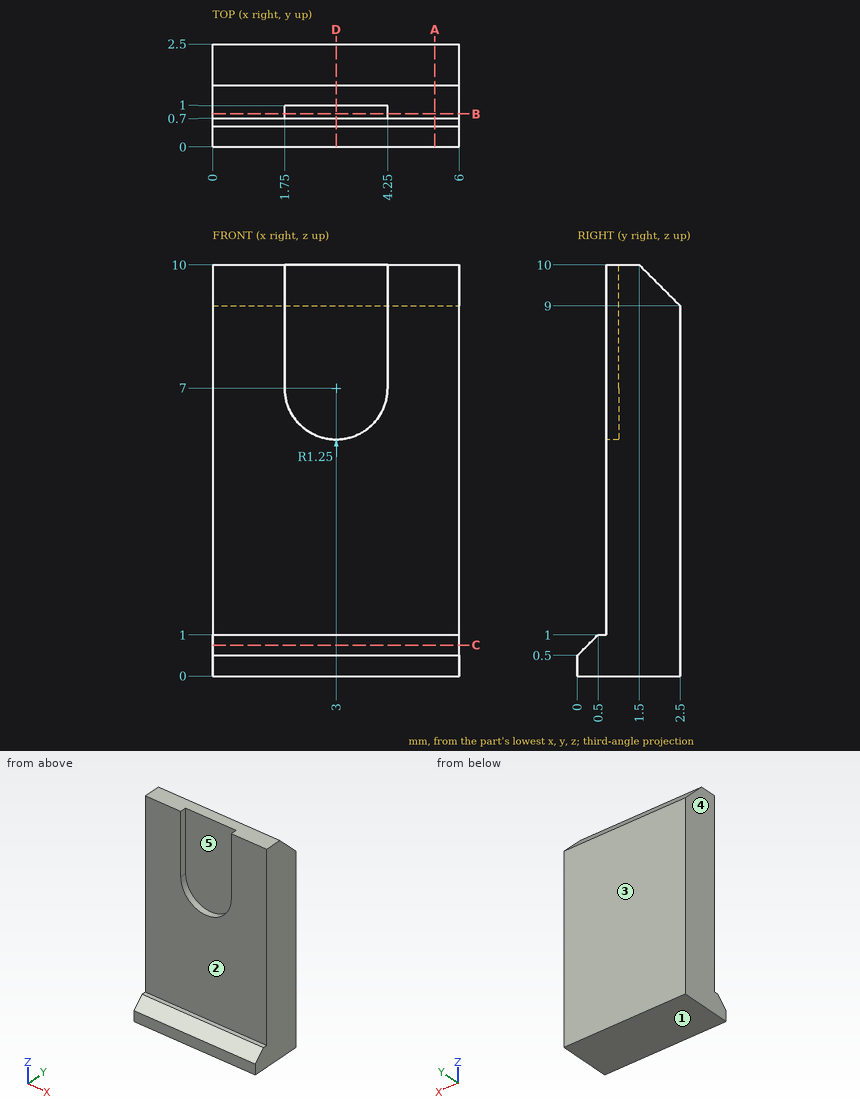
Design review of the part shown in the three views and the two pictorial views. Dimensions are in mm from the part's minimum x, y and z. A direction names the side the tool comes from. Coordinates: 2 decimals unless noted, no trailing zeros. Write each loop counter-clockwise with the first axis right and the second up, starting at its lowest first coordinate (ties: lowest second). Pieces come first, ordered by that corner, then holes.
(1) For pin 1 Ø0.8 at (x, z) = (3, 7) entering from -Y; pin 2 Ø1.5 at (x, z) = (4, 2) entering from -Y; pin 3 Ø1.5 at (x, y) = (3, 1) entering from -Z, all flat-tipped, find the tip position at first contact; note any pin that passes through.
(2) The part is to be moulded in two halves that separate along X. For the marked faces 3, 4 and 5, say which applies: +X half, -X half, draft (parallel to the pull), parting line (faces both ways), or undercut.
(3) Add section B-B on y = 0.8. Give the boundary of the cut face in (x, z).
(4) Add section A-A on x = 5.4. Give the boundary of the cut face in (y, z), then the cut area to 3 significant figures.
(5) Add section C-C on z = 0.75. Give the boundary of the cut face in (x, y).
(6) Add section D-D on x = 3. Give the boundary of the cut face in (y, z).
(7) Tool access review of the marked faces 1 and 2: name each direction out of +Z, -Z, +X, -X, +Y, -Y from which nothing blocks a thin tool from reaching the whole face with its end or side.
(8) Wall thickness on probe 1 along X at (y, z) = (0.75, 9); probe 2 along Y at (x, z) = (2.4, 2.5); probe 3 along Y at (x, z) = (2.3, 6.75): over which ranges is each line inside the solid? List them lowest first.
Answer sheet:
1. pin 1: stops at y = 1
1. pin 2: stops at y = 0.7
1. pin 3: stops at z = 0
2. face 3: draft
2. face 4: -X half
2. face 5: undercut
3. outline: (0, 0) - (6, 0) - (6, 10) - (4.25, 10) - (4.25, 7) arc R1.25 cw to (1.75, 7) - (1.75, 10) - (0, 10) - close
4. outline: (0, 0) - (2.5, 0) - (2.5, 9) - (1.5, 10) - (0.7, 10) - (0.7, 1) - (0.5, 1) - (0, 0.5) - close
4. area: 18.1 mm2
5. outline: (0, 0.25) - (6, 0.25) - (6, 2.5) - (0, 2.5) - close
6. outline: (0, 0) - (2.5, 0) - (2.5, 9) - (1.5, 10) - (1, 10) - (1, 5.75) - (0.7, 5.75) - (0.7, 1) - (0.5, 1) - (0, 0.5) - close
7. face 1: -Z, +X, -X, +Y, -Y
7. face 2: +Z, +X, -X, -Y
8. probe 1: x = 0 to 1.75, 4.25 to 6
8. probe 2: y = 0.7 to 2.5
8. probe 3: y = 1 to 2.5
